```python
from build123d import *

# Parameters (mm, degrees)
F0_R     = 1.5
F0_R_2   = 4.5
F0_R_3   = 3.5
F1_DEPTH = 0.125


with BuildPart() as f1:
    # F0 (on Top) → F1 (new body)
    with BuildSketch(Plane.XY):
        with BuildLine():
            Line((142.75, 122.75), (142.75, 129.75))
            Line((142.75, 129.75), (112.25, 129.75))
            Line((112.25, 129.75), (112.25, 122.75))
            ThreePointArc((112.25, 122.75), (109, 119.5), (105.75, 122.75))
            Line((105.75, 122.75), (105.75, 129.75))
            Line((105.75, 129.75), (76.25, 129.75))
            Line((76.25, 129.75), (76.25, 122.75))
            ThreePointArc((76.25, 122.75), (73, 119.5), (69.75, 122.75))
            Line((69.75, 122.75), (69.75, 129.75))
            Line((69.75, 129.75), (40.25, 129.75))
            Line((40.25, 129.75), (40.25, 122.75))
            ThreePointArc((40.25, 122.75), (37, 119.5), (33.75, 122.75))
            Line((33.75, 122.75), (33.75, 129.75))
            Line((33.75, 129.75), (3, 129.75))
            Line((3, 129.75), (-7, 119.75))
            Line((-7, 119.75), (-7, 89))
            Line((-7, 89), (0, 89))
            ThreePointArc((0, 89), (3.25, 85.75), (0, 82.5))
            Line((0, 82.5), (-7, 82.5))
            Line((-7, 82.5), (-7, 53))
            Line((-7, 53), (0, 53))
            ThreePointArc((0, 53), (3.25, 49.75), (0, 46.5))
            Line((0, 46.5), (-7, 46.5))
            Line((-7, 46.5), (-7, 17))
            Line((-7, 17), (0, 17))
            ThreePointArc((0, 17), (3.25, 13.75), (0, 10.5))
            Line((0, 10.5), (-7, 10.5))
            Line((-7, 10.5), (-7, -20))
            Line((-7, -20), (0, -20))
            ThreePointArc((0, -20), (2.298097, -20.951903), (3.25, -23.25))
            Line((3.25, -23.25), (3.25, -27.75))
            Line((3.25, -27.75), (33.75, -27.75))
            Line((33.75, -27.75), (33.75, -23.25))
            ThreePointArc((33.75, -23.25), (37, -20), (40.25, -23.25))
            Line((40.25, -23.25), (40.25, -27.75))
            Line((40.25, -27.75), (69.75, -27.75))
            Line((69.75, -27.75), (69.75, -23.25))
            ThreePointArc((69.75, -23.25), (73, -20), (76.25, -23.25))
            Line((76.25, -23.25), (76.25, -27.75))
            Line((76.25, -27.75), (105.75, -27.75))
            Line((105.75, -27.75), (105.75, -23.25))
            ThreePointArc((105.75, -23.25), (109, -20), (112.25, -23.25))
            Line((112.25, -23.25), (112.25, -27.75))
            Line((112.25, -27.75), (142.75, -27.75))
            Line((142.75, -27.75), (142.75, -23.25))
            ThreePointArc((142.75, -23.25), (143.701903, -20.951903), (146, -20))
            Line((146, -20), (150.5, -20))
            Line((150.5, -20), (150.5, 10.5))
            Line((150.5, 10.5), (146, 10.5))
            ThreePointArc((146, 10.5), (142.75, 13.75), (146, 17))
            Line((146, 17), (150.5, 17))
            Line((150.5, 17), (150.5, 46.5))
            Line((150.5, 46.5), (146, 46.5))
            ThreePointArc((146, 46.5), (142.75, 49.75), (146, 53))
            Line((146, 53), (150.5, 53))
            Line((150.5, 53), (150.5, 82.5))
            Line((150.5, 82.5), (146, 82.5))
            ThreePointArc((146, 82.5), (142.75, 85.75), (146, 89))
            Line((146, 89), (150.5, 89))
            Line((150.5, 89), (150.5, 119.5))
            Line((150.5, 119.5), (146, 119.5))
            ThreePointArc((146, 119.5), (143.701903, 120.451903), (142.75, 122.75))
        make_face()
        Circle(F0_R, mode=Mode.SUBTRACT)
        with Locations((19, -4.25)):
            Circle(F0_R_2, mode=Mode.SUBTRACT)
        with Locations((55, -4.25)):
            Circle(F0_R_2, mode=Mode.SUBTRACT)
        with Locations((19, 31.75)):
            Circle(F0_R_2, mode=Mode.SUBTRACT)
        with Locations((37, 13.75)):
            Circle(F0_R_3, mode=Mode.SUBTRACT)
        with Locations((37, 49.75)):
            Circle(F0_R_3, mode=Mode.SUBTRACT)
        with Locations((55, 31.75)):
            Circle(F0_R_2, mode=Mode.SUBTRACT)
        with Locations((91, -4.25)):
            Circle(F0_R_2, mode=Mode.SUBTRACT)
        with Locations((127, -4.25)):
            Circle(F0_R_2, mode=Mode.SUBTRACT)
        with Locations((73, 13.75)):
            Circle(F0_R_3, mode=Mode.SUBTRACT)
        with Locations((109, 13.75)):
            Circle(F0_R_3, mode=Mode.SUBTRACT)
        with Locations((91, 31.75)):
            Circle(F0_R_2, mode=Mode.SUBTRACT)
        with Locations((73, 49.75)):
            Circle(F0_R_3, mode=Mode.SUBTRACT)
        with Locations((109, 49.75)):
            Circle(F0_R_3, mode=Mode.SUBTRACT)
        with Locations((127, 31.75)):
            Circle(F0_R_2, mode=Mode.SUBTRACT)
        with Locations((19, 67.75)):
            Circle(F0_R_2, mode=Mode.SUBTRACT)
        with Locations((55, 67.75)):
            Circle(F0_R_2, mode=Mode.SUBTRACT)
        with Locations((37, 85.75)):
            Circle(F0_R_3, mode=Mode.SUBTRACT)
        with Locations((19, 103.75)):
            Circle(F0_R_2, mode=Mode.SUBTRACT)
        with Locations((18.5, 122.8)):
            Circle(F0_R, mode=Mode.SUBTRACT)
        with Locations((55, 103.75)):
            Circle(F0_R_2, mode=Mode.SUBTRACT)
        with Locations((91, 67.75)):
            Circle(F0_R_2, mode=Mode.SUBTRACT)
        with Locations((73, 85.75)):
            Circle(F0_R_3, mode=Mode.SUBTRACT)
        with Locations((109, 85.75)):
            Circle(F0_R_3, mode=Mode.SUBTRACT)
        with Locations((127, 67.75)):
            Circle(F0_R_2, mode=Mode.SUBTRACT)
        with Locations((91, 103.75)):
            Circle(F0_R_2, mode=Mode.SUBTRACT)
        with Locations((127, 103.75)):
            Circle(F0_R_2, mode=Mode.SUBTRACT)
    extrude(amount=F1_DEPTH)


solid = f1.part
```
Can you work these out from the model? Positions are in its coordinate system, mm. Round coordinates to 2 decimals unless told otherwise and drop trailing zeros. Loops run counter-clockwise (first coordinate to the right, second up) from the corner with the lowest first, then second, coordinate; pieces in that order, holes last. Notation, with made-up numbers: M 20,72.25 L 25,72.25 A27 cw 25,91.25 Z; hole C 14,7.25 d3. An arc over 180 degrees is marked long. Answer in a Markdown table with one row per item.
1. If we section it at D-D, the plane z = 0.05: Give the number of separate pieces and of enclosed holes in the cut face, plus the area to 3 significant figures.
Established:
| item | result |
|---|---|
| separate pieces | 1 |
| enclosed holes | 27 |
| area | 22,500 mm² |
2. I'm going to push a flat-ended pin straight in: pin 1 Ø5.5 at (x, y) = (91, 103.75) entering from +Z. Where does the tip first touch, or does it pass through?
Established:
| item | result |
|---|---|
| pin 1 | through |
3. If we section it at B-B, the plane y = -4.25: Please give me the cut outline in (x, z) (3 decimals).
Established:
| item | result |
|---|---|
| outline | M -7,0 L 14.5,0 L 14.5,0.125 L -7,0.125 Z; M 23.5,0 L 50.5,0 L 50.5,0.125 L 23.5,0.125 Z; M 59.5,0 L 86.5,0 L 86.5,0.125 L 59.5,0.125 Z; M 95.5,0 L 122.5,0 L 122.5,0.125 L 95.5,0.125 Z; M 131.5,0 L 150.5,0 L 150.5,0.125 L 131.5,0.125 Z |
4. If we section it at C-C, the plane y = 49.75: Please give me the cut outline in (x, z) (3 decimals).
Established:
| item | result |
|---|---|
| outline | M 3.25,0 L 33.5,0 L 33.5,0.125 L 3.25,0.125 Z; M 40.5,0 L 69.5,0 L 69.5,0.125 L 40.5,0.125 Z; M 76.5,0 L 105.5,0 L 105.5,0.125 L 76.5,0.125 Z; M 112.5,0 L 142.75,0 L 142.75,0.125 L 112.5,0.125 Z |
5. If we section it at A-A, the plane x = 109: Please give me the cut outline in (y, z) (3 decimals), plus the area to 3 significant figures.
Established:
| item | result |
|---|---|
| outline | M -20,0 L 10.25,0 L 10.25,0.125 L -20,0.125 Z; M 17.25,0 L 46.25,0 L 46.25,0.125 L 17.25,0.125 Z; M 53.25,0 L 82.25,0 L 82.25,0.125 L 53.25,0.125 Z; M 89.25,0 L 119.5,0 L 119.5,0.125 L 89.25,0.125 Z |
| area | 14.8 mm² |
6. Please list where this line runs through material, in increasing order: line 1 (Y direction, x = 18.5, z = 0.05). Write a range as from..to.
Established:
| item | result |
|---|---|
| line 1 | -27.75..-8.72, 0.22..27.28, 36.22..63.28, 72.22..99.28, 108.22..121.3, 124.3..129.75 |
